The listing builds one solid part. Answer for the finished solid, in the listing's coordinates (mm). A direction names the side the tool comes from. Give positions to 0.01 mm unless a question says otherwise; leave off trailing zeros. Write each loop counter-clockwise with the first axis right and the second up, starting at its lowest first coordinate (ties: lowest second). Pieces come first, ordered by that corner, then holes. Notation, with made-up numbers: (26.25, 30) - (77.25, 30) arc R18 ccw to (77.25, 46) - close; hole circle Ø5 at (76.5, 20.5). An arc over 180 degrees is marked (long way). One line per question, with ' | ' between items. Start each with the question number.
1. A cutting plane is placed at B-B (z = 7). Determine the outline of the cut face in (x, y).
2. The mould has two halves that part along X. Classify faces 6 (the face through (17, 12, 2)), 7 (the face through (48, 11, 2)), 8 (the face through (1, 7.9, 2)), 9 (the face through (-2, 11, 2)): +X half, -X half, draft (parallel to the pull), parting line (faces both ways), or undercut.
3. A cutting plane is placed at A-A (y = 13). Determine the outline of the cut face in (x, z).
4. Find the intervals of material crossed by L1, parallel to Z at x = 0.5, y = 12; L2, parallel to X at y = 11.25, z = 7.25; L3, parallel to X at y = 11.25, z = 2.25, in increasing order. Write a range as from..to.
5. Given P1, Ø2.5, axis at x = 45.5, z = 7, coming from the +Y side; P2, Ø6, axis at x = 22.5, z = 2.5, coming from the +Y side; P3, Ø4, axis at x = 0.5, z = 7, coming from the -Y side, each flat-ended and moving along its own axis, determine where each tip first touches the part or whether it passes through.
6. A cutting plane is placed at C-C (x = 0.5). Determine the outline of the cut face in (y, z), then the cut area to 3 significant figures.
7. For faces 1 (the face through (38, 11, 0)), 2 (the face through (28.7, 10.26, 0)), 3 (the face through (7, 14.9, 2)), 4 (the face through (45, 7.9, 2)), 5 (the face through (28.55, 10.33, -3.04)), determine the directions among +Z, -Z, +X, -X, +Y, -Y from which every point of the face is accessible in a straight line to the end or side of a thin tool.
8. A cutting plane is placed at D-D (z = -2). Determine the outline of the cut face in (x, y).
```python
from build123d import *
from build123d.topology import SkipClean

# Parameters (mm, degrees)
SKETCH7_R               = 1.5
BOSS_EXTRUDE11_DEPTH    = 10
FILLET1_R               = 20
BOSS_EXTRUDE12_START    = 6
BOSS_EXTRUDE12_DEPTH    = 6
CUT_EXTRUDE1_DEPTH      = 51.142297514
CUT_EXTRUDE1_DEPTH_BACK = 51.142297514
SKETCH10_R              = 1.5


with BuildPart() as part:
    # Sketch7 → Boss-Extrude11 (new body)
    with BuildSketch(Plane.XY):
        Polygon((11, 14.9), (-2, 14.9), (-2, 7.9), (3.598076211, 7.9), (3.598076211, 4.4), (42.4, 4.4), (42.4, 7.9), (48, 7.9), (48, 14.9), (35, 14.9), (29, 14.9), (29, 9.9), (17, 9.9), (17, 14.9), align=None)
        with Locations((8, 10.9)):
            Circle(SKETCH7_R, mode=Mode.SUBTRACT)
        with Locations((38, 10.9)):
            Circle(SKETCH7_R, mode=Mode.SUBTRACT)
    extrude(amount=BOSS_EXTRUDE11_DEPTH)

    # Fillet1
    # the kernel refuses this fillet: 20 mm, written as the material it takes off along each edge
    with BuildSketch(Plane(origin=(42.4, 4.4, -28.256636389), x_dir=(-1.4210854715172548e-12, 1.0, 0), z_dir=(0, 0, 1))) as fillet1_piece_1:
        with BuildLine():
            CenterArc((20, 11.302654555), FILLET1_R, 180, 34.41150867)
            Line((0, 11.302654555), (-0.4, 11.302654555))
            Line((-0.4, 11.302654555), (-0.4, 0))
            Line((-0.4, 0), (0, -0.4))
            ThreePointArc((0, -0.4), (1.75, -0.4), (3.17, -0.226053091))
            Line((3.17, -0.226053091), (3.5, 0))
        make_face()
    extrude(amount=66.513272777, mode=Mode.SUBTRACT)
    with BuildSketch(Plane(origin=(3.598076211, 4.4, -28.256636389), x_dir=(1, 0, 0), z_dir=(0, 0, 1))) as fillet1_piece_2:
        with BuildLine():
            CenterArc((11.302654555, 20), FILLET1_R, 235.58849133, 34.41150867)
            Line((0, 3.5), (-0.226053091, 3.17))
            ThreePointArc((-0.226053091, 3.17), (-0.4, 1.75), (-0.4, 0))
            Line((-0.4, 0), (0, -0.4))
            Line((0, -0.4), (11.302654555, -0.4))
            Line((11.302654555, -0.4), (11.302654555, 0))
        make_face()
    extrude(amount=66.513272777, mode=Mode.SUBTRACT)

    # Sketch9 → Boss-Extrude12 (add)
    with SkipClean():  # the faces are left unmerged after this step: merging them gives an invalid solid
        with BuildSketch(Plane(origin=(0, 0, 0), x_dir=(-1, 0, 0), z_dir=(0, 0, -1)).offset(BOSS_EXTRUDE12_START)):
            with BuildLine():
                Line((-48, 7.9), (-42.4, 7.9))
                ThreePointArc((-42.4, 7.9), (-37.013425228, 5.295026825), (-31.097345445, 4.4))
                Line((-31.097345445, 4.4), (-14.900730767, 4.4))
                ThreePointArc((-14.900730767, 4.4), (-8.984650984, 5.295026825), (-3.598076211, 7.9))
                Line((-3.598076211, 7.9), (2, 7.9))
                Line((2, 7.9), (2, 14.9))
                Line((2, 14.9), (-17, 14.9))
                Line((-17, 14.9), (-17, 11.4))
                ThreePointArc((-17, 11.4), (-17.439339828, 10.339339828), (-18.5, 9.9))
                Line((-18.5, 9.9), (-27.5, 9.9))
                ThreePointArc((-27.5, 9.9), (-28.560660172, 10.339339828), (-29, 11.4))
                Line((-29, 11.4), (-29, 14.9))
                Line((-29, 14.9), (-48, 14.9))
                Line((-48, 14.9), (-48, 7.9))
            make_face()
        extrude(amount=-BOSS_EXTRUDE12_DEPTH)

    # Sketch10 → Cut-Extrude1 (cut, two sides: drawn at the far end of the back side and taken through both)
    with SkipClean():  # the faces are left unmerged after this step: merging them gives an invalid solid
        with BuildSketch(Plane(origin=(0, 14.9, 0), x_dir=(1, 0, 0), z_dir=(0, 1, 0)).offset(-CUT_EXTRUDE1_DEPTH_BACK)):
            with Locations(Location((0.5, -7, 0), (0, 0, 180))):
                Circle(SKETCH10_R)
            with Locations(Location((0.5, 3, 0), (0, 0, 180))):
                Circle(SKETCH10_R)
            with Locations(Location((45.5, -7, 0), (0, 0, 180))):
                Circle(SKETCH10_R)
            with Locations(Location((45.5, 3, 0), (0, 0, 180))):
                Circle(SKETCH10_R)
        extrude(amount=CUT_EXTRUDE1_DEPTH + CUT_EXTRUDE1_DEPTH_BACK, mode=Mode.SUBTRACT)


solid = part.part
```
Determined:
1) outline: (-2, 7.9) - (-1, 7.9) - (-1, 14.9) - (-2, 14.9) - close; (2, 7.9) - (3.6, 7.9) arc R20 ccw to (14.9, 4.4) - (31.1, 4.4) arc R20 ccw to (42.4, 7.9) - (44, 7.9) - (44, 14.9) - (29, 14.9) - (29, 9.9) - (17, 9.9) - (17, 14.9) - (2, 14.9) - close; (47, 7.9) - (48, 7.9) - (48, 14.9) - (47, 14.9) - close; hole circle Ø3 at (8, 10.9); hole circle Ø3 at (38, 10.9)
2) face 6: undercut | face 7: +X half | face 8: draft | face 9: -X half
3) outline: (-2, -6) - (17, -6) - (17, 10) - (-2, 10) - close; (29, -6) - (48, -6) - (48, 10) - (29, 10) - close; hole circle Ø3 at (0.5, -3); hole circle Ø3 at (0.5, 7); hole circle Ø3 at (45.5, -3); hole circle Ø3 at (45.5, 7)
4) L1: -6..-4.5, -1.5..5.5, 8.5..10 | L2: -2..-0.98, 1.98..6.54, 9.46..17, 29..36.54, 39.46..44.02, 46.98..48 | L3: -2..6.54, 9.46..17, 29..36.54, 39.46..48
5) P1: through | P2: y = 9.9 | P3: y = 7.9
6) outline: (7.9, -6) - (14.9, -6) - (14.9, -4.5) - (7.9, -4.5) - close; (7.9, -1.5) - (14.9, -1.5) - (14.9, 5.5) - (7.9, 5.5) - close; (7.9, 8.5) - (14.9, 8.5) - (14.9, 10) - (7.9, 10) - close | area: 70.0 mm2
7) face 1: +Z | face 2: +Z, +Y | face 3: +Z, -Z, +X, -X, +Y | face 4: +Z, -Z, +X, -Y | face 5: +Z, -Z, +Y
8) outline: (-2, 7.9) - (-0.62, 7.9) - (-0.62, 14.9) - (-2, 14.9) - close; (1.62, 7.9) - (3.6, 7.9) arc R20 ccw to (14.9, 4.4) - (31.1, 4.4) arc R20 ccw to (42.4, 7.9) - (44.38, 7.9) - (44.38, 14.9) - (29, 14.9) - (29, 11.4) arc R1.5 cw to (27.5, 9.9) - (18.5, 9.9) arc R1.5 cw to (17, 11.4) - (17, 14.9) - (1.62, 14.9) - close; (46.62, 7.9) - (48, 7.9) - (48, 14.9) - (46.62, 14.9) - close
